from build123d import *

# Parameters (mm, degrees)
F0_W      = 345
F0_H      = 106
F1_DEPTH  = 2
F2_SIZE   = 10
F3_SIZE   = 10
F4_R      = 1.75
F5_DEPTH  = 25
F6_R      = 15
F6_W      = 22
F6_H      = 8
F7_DEPTH  = 25
F9_R      = 6.5
F9_R_2    = 11.5
F9_R_3    = 3.2
F10_DEPTH = 25
F6_R_2    = 4.85
F11_DEPTH = 25


# Not quite as in the source:
# - a feature names something its author has since deleted; it is built from what else it names


with BuildPart() as f1:
    # F0 (on Front) → F1 (new body)
    with BuildSketch(Plane.XZ):
        with Locations((46.1619326359, 29.679378029)):
            Rectangle(F0_W, F0_H)
    extrude(amount=F1_DEPTH)

    # F2
    f2_edges = [f1.edges().sort_by_distance(p)[0] for p in [
        (-126.338067, -1, 82.679378),
    ]]
    chamfer(f2_edges, length=F2_SIZE)

    # F3
    f3_edges = [f1.edges().sort_by_distance(p)[0] for p in [
        (-126.338067, -1, -23.320622),
        (218.661933, -1, -23.320622),
        (218.661933, -1, 82.679378),
    ]]
    chamfer(f3_edges, length=F3_SIZE)

    # F4 (on face) → F5 (cut)
    with BuildSketch(Plane.XZ.offset(2)):
        with Locations((-121.3380673641, 45.679378029)):
            Circle(F4_R)
        with Locations((-120.3380673641, 13.679378029)):
            Circle(F4_R)
        with Locations((212.6619326359, 45.679378029)):
            Circle(F4_R)
        with Locations((212.6619326359, 13.679378029)):
            Circle(F4_R)
    extrude(amount=-F5_DEPTH, mode=Mode.SUBTRACT)

    # F6 (on face) → F7 (cut)
    with BuildSketch(Plane.XZ.offset(2)):
        with Locations((-66.3380673641, 29.679378029)):
            Circle(F6_R)
        with Locations((-6.3380673641, 29.679378029)):
            Circle(F6_R)
        with Locations((53.6619326359, 29.679378029)):
            Rectangle(F6_W, F6_H)
    extrude(amount=-F7_DEPTH, mode=Mode.SUBTRACT)

    # F9 (on face) → F10 (cut)
    with BuildSketch(Plane.XZ.offset(2)):
        with Locations((188.6619326359, 52.679378029)):
            Circle(F9_R)
        with Locations((153.6619326359, 29.679378029)):
            Circle(F9_R_2)
        with Locations((188.6619326359, 16.679378029)):
            Circle(F9_R_3)
    extrude(amount=-F10_DEPTH, mode=Mode.SUBTRACT)

    # F6 (on face) → F11 (cut)
    with BuildSketch(Plane.XZ.offset(2)):
        with Locations((-66.3380673641, 29.679378029)):
            Circle(F6_R)
        with Locations((-6.3380673641, 29.679378029)):
            Circle(F6_R)
        with Locations((53.6619326359, 29.679378029)):
            Rectangle(F6_W, F6_H)
        with Locations((113.6619326359, 29.679378029)):
            Circle(F6_R_2)
    extrude(amount=-F11_DEPTH, mode=Mode.SUBTRACT)


solid = f1.part
Could you check a few things on this model? Use its own coordinates, in mm. Coordinates: 2 decimals unless noted, no trailing zeros. Order: outer loops, then holes, each group sorted by start corner. A loop starts at its lowest first (then second) coordinate and runs counter-clockwise, first axis right, second up. Notation, with made-up numbers: (61, 68.25) - (78, 68.25) arc R12 ccw to (78, 76.25) - close; hole circle Ø9 at (41, 24). An arc over 180 degrees is marked (long way). Answer in a Markdown table with one row per item. Add a question column.
(1) If we section it at B-B, the plane y = -0.4: State how many separate pieces and enclosed holes the cut face has, then the cut area to 3 significant figures.
(2) If we section it at C-C, the plane x = -56.5: Please give me the cut outline in (y, z).
(3) Will these pins go through, and if not, where does the flat tip stop? pin 1 (3 mm diameter, centred on x = -120.34, z = 13.68, fed in from +Y); pin 2 (4.5 mm diameter, centred on x = 212.66, z = 45.68, fed in from -Y).
(4) I need wall thicknesses on L1, parallel to Z at x = 62, y = -1.85; L2, parallel to X at y = -1.9, z = 42; L3, parallel to X at y = -0.7, z = 53. Which ranges of each line are inside material? Lowest first, please.
(5) If we section it at A-A, the plane x = 154.5: Please give me the cut outline in (y, z).
(6) If we mould it in two halves opening along X, with no side actions, what happens to faces 1 (the face through (44, 0, 42)), 2 (the face through (-8.29, -1.01, 44.55)), 3 (the face through (213.73, -0.99, -18.25))? For each: released by +X, released by -X, zero draft, split by the parting line, or undercut.
Results are:
| question | item | result |
|---|---|---|
| 1 | separate pieces | 1 |
| 1 | enclosed holes | 11 |
| 1 | area | 34,100 mm2 |
| 2 | outline | (-2, -23.32) - (0, -23.32) - (0, 18.36) - (-2, 18.36) - close; (-2, 41) - (0, 41) - (0, 82.68) - (-2, 82.68) - close |
| 3 | pin 1 | passes through |
| 3 | pin 2 | stops at y = -2 |
| 4 | L1 | z = -23.32 to 25.68, 33.68 to 82.68 |
| 4 | L2 | x = -126.34 to -74.89, -57.78 to -14.89, 2.22 to 218.66 |
| 4 | L3 | x = -126.34 to 182.17, 195.15 to 218.66 |
| 5 | outline | (-2, -23.32) - (0, -23.32) - (0, 18.21) - (-2, 18.21) - close; (-2, 41.15) - (0, 41.15) - (0, 82.68) - (-2, 82.68) - close |
| 6 | face 1 | zero draft |
| 6 | face 2 | undercut |
| 6 | face 3 | released by +X |
